Geometry: final body of the model. Coordinates: model frame, mm. A direction names the side the tool comes from. Coordinates: 2 decimals unless noted, no trailing zeros. Loops run counter-clockwise (first coordinate to the right, second up) from the corner with the lowest first, then second, coordinate; pieces in that order, holes last. Notation, with made-up numbers: (-33, 80.25) - (-5, 80.25) arc R22 cw to (-5, 115.25) - close; hole circle Ø3 at (51.5, 29). An arc over 180 degrees is marked (long way). Put each result on its own line as item: value. Start each with the question number.
1) Section B-B on z = 7. Output: boundary loops of the cut face in (x, y), and give its area (3 significant figures).
2) Draft query along X for faces 3 (the conical face through (0, 0, -15)), 4 (the flat face through (-1, 1, 0)), 5 (the cylindrical face through (-0.738, -2.345, 24.93)). Return one class per face: +X half, -X half, draft (parallel to the pull), parting line (faces both ways), or undercut.
3) Section A-A on z = -4. Output: boundary loops of the cut face in (x, y), and give its area (3 significant figures).
4) Material intervals for line 1 along Y through (x, z) = (0, 27); line 2 along Z through (x, y) = (2.5, 0); line 3 along X through (y, z) = (2, 3), sorted ascending. Write a range as from..to.
5) Reachability of faces 1 (the cylindrical face through (-0.867, 3.905, 15.297)), 2 (the cylindrical face through (0, 1, -7)) from +Z, -Z, +X, -X, +Y, -Y: full face, straight path, thin tool, end or side. Return the list, or none.
6) Contact query for flat-ended pins moving along their axis: pin 1 Ø1 at (x, z) = (-2.5, 15) entering from +Y; pin 2 Ø3 at (x, y) = (1.5, -0.5) entering from -Z; pin 3 Ø4 at (y, z) = (2, -8.5) entering from -X. Output: stop coordinate, or through.
Autodesk Inventor part; units mm, degrees
ref_plane "YZ Plane" through (0, 0, 0) normal (1, 0, 0) x (0, 1, 0)
ref_plane "XZ Plane" through (0, 0, 0) normal (0, 1, 0) x (-1, 0, 0)
ref_plane "XY Plane" through (0, 0, 0) normal (0, 0, 1) x (1, 0, 0)
sketch "Sketch1" plane through (0, 0, 0) normal (0, 0, 1) x (1, 0, 0)
  circle A0 centre (0, 0) radius 4
  dimension "d0" = 8
extrude "Extrusion1" add sketch "Sketch1" along normal blind 30
sketch "Sketch2" plane through (0, 0, 0) normal (0, 0, -1) x (-1, 0, 0)
  circle A0 centre (0, 0) radius 1
  dimension "d3" = 2
extrude "Extrusion2" add sketch "Sketch2" along normal blind 15
chamfer "Chamfer1" distance 1 angle 45 1 edges at (1, 0, -15)
chamfer "Chamfer2" distance 1 angle 45 1 edges at (-4, 0, 0)
sketch "Sketch3" plane through (0, 0, 30) normal (0, 0, 1) x (1, 0, 0)
  point P0 (0, 0)
  point P1 (0, 0)
hole "Hole1" at (0, 0, 30) direction (0, 0, -1) diameter 4.917 depth 10 tip angle 118
properties part number "top"
Answer block:
1. outline: circle Ø8 at (0, 0)
1. area: 50.3 mm²
2. face 3: parting line
2. face 4: draft
2. face 5: undercut
3. outline: circle Ø2 at (0, 0)
3. area: 3.14 mm²
4. line 1: y = -4..-2.46, 2.46..4
4. line 2: z = 0..30
4. line 3: x = -3.46..3.46
5. face 1: +Z, -Z
5. face 2: -Z
6. pin 1: stops at y = 3.46
6. pin 2: stops at z = -14.92
6. pin 3: stops at x = -1
